```python
from build123d import *

# Parameters (mm, degrees)
SKETCH1_R           = 2.125
SKETCH1_R_2         = 2.5527
BOSS_EXTRUDE1_DEPTH = 6.35
FILLET1_R           = 5.08


with BuildPart() as part:
    # Sketch1 → Boss-Extrude1 (new body)
    with BuildSketch(Plane.XY):
        with BuildLine():
            Line((31.499999992, 0), (31.499999992, 84.3))
            ThreePointArc((31.499999992, 84.3), (0, 115.799999992), (-31.499999992, 84.3))
            Line((-31.499999992, 84.3), (-31.499999992, 0))
            Line((-31.499999992, 0), (31.499999992, 0))
        make_face()
        with Locations((15.556349186, 68.743650814)):
            Circle(SKETCH1_R, mode=Mode.SUBTRACT)
        with Locations((19.05, 12.7)):
            Circle(SKETCH1_R_2, mode=Mode.SUBTRACT)
        with Locations((0, 12.7)):
            Circle(SKETCH1_R_2, mode=Mode.SUBTRACT)
        with Locations((0, 38.1)):
            Circle(SKETCH1_R_2, mode=Mode.SUBTRACT)
        with Locations((19.05, 38.1)):
            Circle(SKETCH1_R_2, mode=Mode.SUBTRACT)
        with Locations((-19.05, 12.7)):
            Circle(SKETCH1_R_2, mode=Mode.SUBTRACT)
        with Locations((-19.05, 38.1)):
            Circle(SKETCH1_R_2, mode=Mode.SUBTRACT)
        with BuildLine():
            ThreePointArc((15.556349186, 101.981349186), (12.082063653, 101.799269597), (8.645843119, 101.255025731))
            ThreePointArc((8.645843119, 101.255025731), (7.00909181, 98.734649736), (9.529467805, 97.097898427))
            ThreePointArc((9.529467805, 97.097898427), (12.526309622, 97.572551541), (15.556349186, 97.731349186))
            ThreePointArc((15.556349186, 97.731349186), (17.681349186, 99.856349186), (15.556349186, 101.981349186))
        make_face(mode=Mode.SUBTRACT)
        with BuildLine():
            ThreePointArc((-17.681349186, 68.743650814), (-17.499269597, 65.26936528), (-16.955025731, 61.833144746))
            ThreePointArc((-16.955025731, 61.833144746), (-14.434649736, 60.196393438), (-12.797898427, 62.716769432))
            ThreePointArc((-12.797898427, 62.716769432), (-13.272551541, 65.713611249), (-13.431349186, 68.743650814))
            ThreePointArc((-13.431349186, 68.743650814), (-15.556349186, 70.868650814), (-17.681349186, 68.743650814))
        make_face(mode=Mode.SUBTRACT)
        with BuildLine():
            ThreePointArc((-17.058951096, 101.358951096), (-20.289508286, 97.771053851), (-23.12733076, 93.865126304))
            ThreePointArc((-23.12733076, 93.865126304), (-22.502513753, 90.925593398), (-19.562980847, 91.550410405))
            ThreePointArc((-19.562980847, 91.550410405), (-16.98663795, 95.096442189), (-14.053747276, 98.353747276))
            ThreePointArc((-14.053747276, 98.353747276), (-14.053747276, 101.358951096), (-17.058951096, 101.358951096))
        make_face(mode=Mode.SUBTRACT)
        with BuildLine():
            ThreePointArc((-4.242640687, 88.542640687), (-6.203737735, 86.364621763), (-7.926426716, 83.993543794))
            ThreePointArc((-7.926426716, 83.993543794), (-6.162237519, 75.693686177), (2.137620099, 77.457875374))
            ThreePointArc((2.137620099, 77.457875374), (3.122013803, 78.812777071), (4.242640687, 80.057359313))
            ThreePointArc((4.242640687, 80.057359313), (4.242640687, 88.542640687), (-4.242640687, 88.542640687))
        make_face(mode=Mode.SUBTRACT)
    extrude(amount=BOSS_EXTRUDE1_DEPTH)

    # Fillet1
    fillet1_edges = [part.edges().sort_by_distance(p)[0] for p in [
        (31.499999992, 0, 3.175),
        (-31.499999992, 0, 3.175),
    ]]
    fillet(fillet1_edges, radius=FILLET1_R)


solid = part.part
```
Input: part model. Units: mm. Frame: model coordinates. A direction names the side the tool comes from. Round coordinates to 2 decimals unless told otherwise and drop trailing zeros. Order: outer loops, then holes, each group sorted by start corner. A loop starts at its lowest first (then second) coordinate and runs counter-clockwise, first axis right, second up. Notation, with made-up numbers: (29.5, 62) - (65.5, 62) arc R24 ccw to (65.5, 89) - close; hole circle Ø10 at (21, 39.5). An arc over 180 degrees is marked (long way). Answer in a Markdown table with one row per item.
Item 1: Section query D-D (x = 19.05). Return the cut outline in (y, z).
Model answer:
| item | result |
|---|---|
| outline | (0, 0) - (10.15, 0) - (10.15, 6.35) - (0, 6.35) - close; (15.25, 0) - (35.55, 0) - (35.55, 6.35) - (15.25, 6.35) - close; (40.65, 0) - (109.39, 0) - (109.39, 6.35) - (40.65, 6.35) - close |
Item 2: Line query: line 1 (X direction, y = 69, z = 2); line 2 (Y direction, x = -20, z = 2.5); line 3 (X direction, y = 39.5, z = 5.75). Output: solid intervals per line, ascending.
Model answer:
| item | result |
|---|---|
| line 1 | x = -31.5 to -17.67, -13.45 to 13.45, 17.67 to 31.5 |
| line 2 | y = 0 to 10.33, 15.07 to 35.73, 40.47 to 91.06, 98.12 to 108.64 |
| line 3 | x = -31.5 to -21.18, -16.92 to -2.13, 2.13 to 16.92, 21.18 to 31.5 |
Item 3: Section query A-A (y = 38.1). Return the cut outline in (x, z), then the cut area to 3 significant figures.
Model answer:
| item | result |
|---|---|
| outline | (-31.5, 0) - (-21.6, 0) - (-21.6, 6.35) - (-31.5, 6.35) - close; (-16.5, 0) - (-2.55, 0) - (-2.55, 6.35) - (-16.5, 6.35) - close; (2.55, 0) - (16.5, 0) - (16.5, 6.35) - (2.55, 6.35) - close; (21.6, 0) - (31.5, 0) - (31.5, 6.35) - (21.6, 6.35) - close |
| area | 303 mm² |
Item 4: Mould query, pull axis X, two halves, no side actions, for faces 3 (the cylindrical face through (-13.268, 65.671, 3.131)), 4 (the cylindrical face through (15.28, 70.85, 3.13)), 5 (the flat face through (31.5, 44, 3)), 6 (the cylindrical face through (0.693, 115.792, 3.131)). Classes: released by +X, released by -X, zero draft, split by the parting line, or undercut.
Model answer:
| item | result |
|---|---|
| face 3 | undercut |
| face 4 | undercut |
| face 5 | released by +X |
| face 6 | split by the parting line |
Item 5: Reachability of faces 1 (the cylindrical face through (30.051, 1.528, 3.219)), 2 (the cylindrical face through (17.68, 99.81, 3.13)) from +Z, -Z, +X, -X, +Y, -Y: full face, straight path, thin tool, end or side. Return the list, or none.
Model answer:
| item | result |
|---|---|
| face 1 | +Z, -Z, +X, -Y |
| face 2 | +Z, -Z |
Item 6: Section query C-C (z = 4.25). Give the number of separate pieces and of enclosed holes in the cut face, then the cut area to 3 significant figures.
Model answer:
| item | result |
|---|---|
| separate pieces | 1 |
| enclosed holes | 11 |
| area | 6,420 mm² |
Item 7: Section query B-B (x = 0). Return the cut outline in (y, z), then the cut area to 3 significant figures.
Model answer:
| item | result |
|---|---|
| outline | (0, 0) - (10.15, 0) - (10.15, 6.35) - (0, 6.35) - close; (15.25, 0) - (35.55, 0) - (35.55, 6.35) - (15.25, 6.35) - close; (40.65, 0) - (75.47, 0) - (75.47, 6.35) - (40.65, 6.35) - close; (90.3, 0) - (115.8, 0) - (115.8, 6.35) - (90.3, 6.35) - close |
| area | 576 mm² |
Item 8: Pin query (flat end, axial travel): pin 1 (4 mm diameter, centred on x = 0, y = 38.1, fed in from +Z). Return the tip coordinate at first contact, or that it passes through.
Model answer:
| item | result |
|---|---|
| pin 1 | passes through |
